from build123d import *

# Parameters (mm, degrees)
SCHIZZO1_R                   = 1.75
ESTRUSIONE_ESTRUSIONE1_DEPTH = 4
TAGLIO_ESTRUSIONE1_DEPTH     = 14.597426227
RACCORDO1_R                  = 1


with BuildPart() as part:
    # Schizzo1 → Estrusione-Estrusione1 (new body)
    with BuildSketch(Plane(origin=(0, 0, 0), x_dir=(1, 0, 0), z_dir=(0, 1, 0))):
        with BuildLine():
            Line((-4.15, 0), (-4.15, 10))
            Line((-4.15, 10), (4.15, 10))
            Line((4.15, 10), (4.15, 0))
            ThreePointArc((4.15, 0), (0, -4.15), (-4.15, 0))
        make_face()
        with Locations(Location((0, 0, 0), (0, 0, 270))):
            Circle(SCHIZZO1_R, mode=Mode.SUBTRACT)
    extrude(amount=ESTRUSIONE_ESTRUSIONE1_DEPTH)

    # Schizzo2 → Taglio-Estrusione1 (cut, through all)
    with BuildSketch(Plane(origin=(4.15, 0, 0), x_dir=(0, 0, -1), z_dir=(1, 0, 0))):
        Polygon((10, 2), (10, 4), (3, 4), align=None)
    extrude(amount=-TAGLIO_ESTRUSIONE1_DEPTH, mode=Mode.SUBTRACT)

    # Raccordo1
    raccordo1_edges = [part.edges().sort_by_distance(p)[0] for p in [
        (-4.15, 1, -10),
        (4.15, 1, -10),
    ]]
    fillet(raccordo1_edges, radius=RACCORDO1_R)


solid = part.part
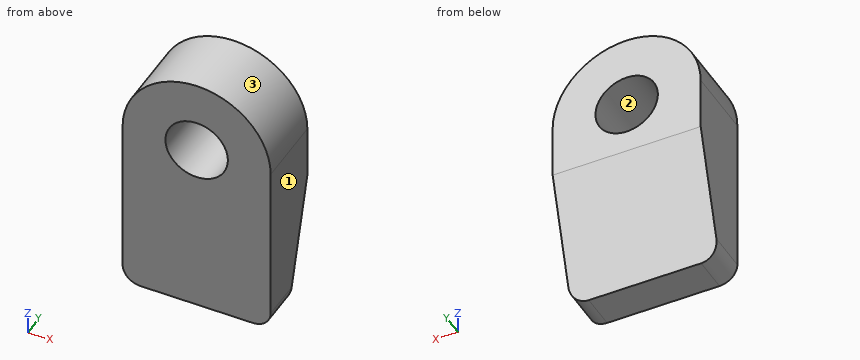
Geometry check sheet. Reference: the model listing, model coordinates, mm. Face numbers are marked on the shaded views. Round coordinates to 2 decimals unless told otherwise and drop trailing zeros. Order: outer loops, then holes, each group sorted by start corner. A loop starts at its lowest first (then second) coordinate and runs counter-clockwise, first axis right, second up. Notation, with made-up numbers: M -19,-7 L 38,-7 A21 ccw 38,13 Z; hole C -34.5,11.25 d7. An arc over 180 degrees is marked long. Write each question's results on one line, items separated by ' | '. Start each with the question number.
1. Draft check along Z on the marked faces 1, 2 and 3. Enter one of: pulls with the +Z half, pulls with the -Z half, needs draft (parallel to the pull), parting line crosses it, or undercut.
2. Cross-section at B-B on y = 1.6. Record the boundary of the cut face in (x, z), plus the area to 3 significant figures.
3. Material ranges on L1, parallel to Y at x = -1.25, z = -9; L2, parallel to X at y = 3.6, z = 0.75; L3, parallel to Z at x = -0.5, y = 1, recorded low to high. Write a range as from..to.
4. Cross-section at D-D on y = 3. Record the boundary of the cut face in (x, z).
5. Go/stop test with flat-tipped pins: P1, Ø1, axis at x = -2, z = -5, coming from the +Y side; P2, Ø4, axis at x = -1, z = -1, coming from the +Y side; P3, Ø1.5, axis at x = -1, y = 1, coming from the +Z side; P4, Ø3, axis at x = 0, z = 0, coming from the -Y side. Record where each tip stops, or that it passes through.
6. Cross-section at A-A on x = 0. Record the boundary of the cut face in (y, z).
7. Cross-section at C-C on z = 0.25. Record the boundary of the cut face in (x, y).
Resolved:
1) face 1: needs draft | face 2: undercut | face 3: pulls with the +Z half
2) outline: M -4.15,-9 A1 ccw -3.15,-10 L 3.15,-10 A1 ccw 4.15,-9 L 4.15,0 A4.15 ccw -4.15,0 Z; hole C 0,0 d3.5 | area: 100 mm2
3) L1: 0..2.29 | L2: -4.08..-1.58, 1.58..4.08 | L3: -10..-1.68, 1.68..4.12
4) outline: M -4.15,-6.5 L 4.15,-6.5 L 4.15,0 A4.15 ccw -4.15,0 Z; hole C 0,0 d3.5
5) P1: y = 3.57 | P2: y = 4 | P3: z = 4.14 | P4: through
6) outline: M 0,-10 L 2,-10 L 4,-3 L 4,-1.75 L 0,-1.75 Z; M 0,1.75 L 4,1.75 L 4,4.15 L 0,4.15 Z
7) outline: M -4.14,0 L -1.73,0 L -1.73,4 L -4.14,4 Z; M 1.73,0 L 4.14,0 L 4.14,4 L 1.73,4 Z
